Geometry: final body of the model. Coordinates: model frame, mm. Round coordinates to 2 decimals unless told otherwise and drop trailing zeros. Write each loop counter-clockwise with the first axis right and the second up, starting at its lowest first coordinate (ties: lowest second). Pieces come first, ordered by that corner, then holes. Notation, with made-up numbers: M -23,40.25 L 18,40.25 A19 ccw 18,72.25 Z; hole C 37.25,68 d1. An arc over 180 degrees is marked long. Use one line per item in the form item = value. Start each with the question number.
Item 1: Ray query, probe 1 along X at (y, z) = (147, 2.7); probe 2 along Y at (x, z) = (18, 1.3); probe 3 along X at (y, z) = (255, 0.45). Return the intervals inside material, ascending.
Item 2: Section query B-B (x = -15.5). State how many separate pieces and enclosed holes the cut face has, and give its area (3 significant figures).
Item 3: Section query A-A (x = -0.5). Return loops of the section in (y, z) (3 decimals).
from build123d import *

# Parameters (mm, degrees)
BOSS_EXTRUDE1_DEPTH = 3.175
FILLET1_R           = 12.7


with BuildPart() as part:
    # Sketch1 → Boss-Extrude1 (new body)
    with BuildSketch(Plane.XY):
        with BuildLine():
            Line((34.35, 6.35), (0, 6.35))
            Line((0, 6.35), (0, 0))
            Line((0, 0), (40.7, 0))
            Line((40.7, 0), (40.7, 147.32))
            Line((40.7, 147.32), (3.175, 147.32))
            add(Edge.make_bspline(
                [(34.35, 6.35), (45.415498484, 56.545116153), (2.852403288, 97.787684056), (3.175, 147.32)],
                knots=[0, 0, 0, 0, 1, 1, 1, 1], degree=3))
        make_face()
    extrude(amount=BOSS_EXTRUDE1_DEPTH)

    # Mirror1: part across plane


with BuildPart() as part_1:
    add(part.part)
    add(part.part.mirror(Plane(origin=(0, 0, 3.175), x_dir=(0, 0, 1), z_dir=(-1, 0, 0))))

    # Mirror2: part across plane


with BuildPart() as part_2:
    add(part_1.part)
    add(part_1.part.mirror(Plane(origin=(-3.175, 147.32, 3.175), x_dir=(0, 0, 1), z_dir=(0, 1, 0))))

    # Fillet1
    fillet1_edges = [part_2.edges().sort_by_distance(p)[0] for p in [
        (34.35, 6.35, 1.5875),
        (-34.35, 6.35, 1.5875),
        (34.35, 288.29, 1.5875),
        (-34.35, 288.29, 1.5875),
    ]]
    fillet(fillet1_edges, radius=FILLET1_R)


solid = part_2.part
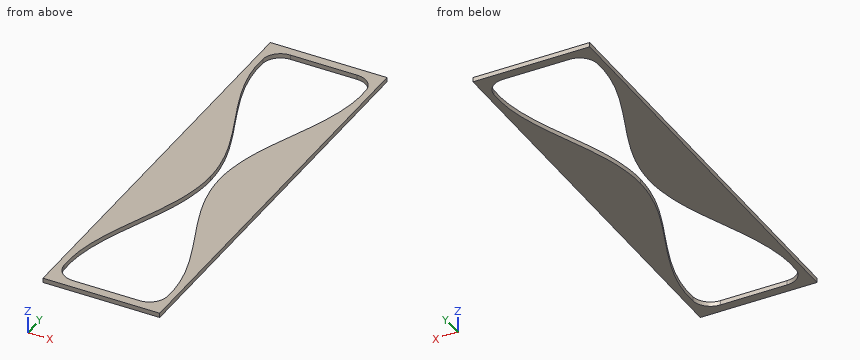
Working result:
q1.probe_1 = -40.7 to -3.17, 3.17 to 40.7
q1.probe_2 = 0 to 6.35, 88.78 to 205.86, 288.29 to 294.64
q1.probe_3 = -40.7 to -34.67, 34.67 to 40.7
q2.separate_pieces = 3
q2.enclosed_holes = 0
q2.area = 373 mm²
q3.outline = M 0,0 L 6.35,0 L 6.35,3.175 L 0,3.175 Z; M 288.29,0 L 294.64,0 L 294.64,3.175 L 288.29,3.175 Z
